Autodesk Inventor part; units mm, degrees
ref_plane "YZ Plane" through (0, 0, 0) normal (1, 0, 0) x (0, 1, 0)
ref_plane "XZ Plane" through (0, 0, 0) normal (0, 1, 0) x (-1, 0, 0)
ref_plane "XY Plane" through (0, 0, 0) normal (0, 0, 1) x (1, 0, 0)
sketch "Sketch1" plane through (0, 0, 0) normal (0, 0, 1) x (1, 0, 0)
  line L0 (0, 0) -> (14, 0)
  line L1 (14, 0) -> (14, -14)
  line L2 (14, -14) -> (0, -14)
  line L3 (0, -14) -> (0, 0)
  dimension "d0" = 14
  dimension "d1" = 14
extrude "Extrusion1" add sketch "Sketch1" against normal blind 22
sketch "Sketch2" plane through (0, 0, 0) normal (0, 0, 1) x (1, 0, 0)
  line L0 (2, -2) -> (12, -2)
  line L1 (12, -2) -> (12, -22)
  line L2 (12, -22) -> (2, -22)
  line L3 (2, -22) -> (2, -2)
  point P0 (0, 0)
  dimension "d4" = 10
  dimension "d5" = 20
extrude "Extrusion2" cut sketch "Sketch2" against normal blind 20
sketch "Sketch5" plane through (0, -14, 0) normal (-1, 0, 0) x (0, 0, 1)
  line L0 (-13, 12) -> (-18, 12)
  line L1 (-18, 12) -> (-18, -8)
  line L2 (-18, -8) -> (-13, -8)
  line L3 (-13, -8) -> (-13, 12)
  point P0 (0, 14)
  dimension "d11" = 5
  dimension "d12" = 20
extrude "Extrusion4" cut sketch "Sketch5" against normal blind 2
properties part number "housing_v03"
Read the model definition and answer for the solid it produces. Units are mm, in the model's axes. A direction names the side the tool comes from. Round coordinates to 2 decimals unless told otherwise and drop trailing zeros. Write each loop counter-clockwise with the first axis right and the second up, starting at its lowest first coordinate (ties: lowest second). Pieces come first, ordered by that corner, then holes. Notation, with made-up numbers: (45.5, 70.5) - (51.5, 70.5) arc R27 cw to (51.5, 102.5) - close; hole circle Ø2 at (-2, -21). An arc over 180 degrees is marked (long way). Use CSV: the item, a comma, the result in double quotes.
Q1. This flat-tipped pin is pushed along its axis until it touches: pin 1 Ø3.5 at (x, z) = (7.5, -9) entering from -Y. Where does it stop, or does it pass through?
Values:
pin 1,"stops at y = -2"
Q2. A tool of negligible diameter and unlimited length cuts with its end or side. For faces 1 (the flat face through (1, -8, -13)), 2 (the flat face through (14, -7, -11)), 3 (the flat face through (2, -8, -6)), from which of +Z, -Z, +X, -X, +Y, -Y can it reach the whole face along a straight path? Write none if from no direction.
Values:
face 1,"-X, -Y"
face 2,"+Z, -Z, +X, +Y, -Y"
face 3,"+Z, -Y"
Q3. Find section C-C, the plane x = 8. Write down the section's boundary in (y, z), then the cut area to 3 significant figures.
Values:
outline,"(-14, -22) - (0, -22) - (0, 0) - (-2, 0) - (-2, -20) - (-14, -20) - close"
area,"68.0 mm²"
Q4. Find section D-D, the plane z = -14. Write down the section's boundary in (x, y), then the cut area to 3 significant figures.
Values:
outline,"(0, -2) - (12, -2) - (12, -14) - (14, -14) - (14, 0) - (0, 0) - close"
area,"52.0 mm²"
Q5. Find section B-B, the plane z = -5.5. Write down the section's boundary in (x, y), then the cut area to 3 significant figures.
Values:
outline,"(0, -14) - (2, -14) - (2, -2) - (12, -2) - (12, -14) - (14, -14) - (14, 0) - (0, 0) - close"
area,"76.0 mm²"
Q6. Find section A-A, the plane y = -3.25. Write down the section's boundary in (x, z).
Values:
outline,"(0, -22) - (14, -22) - (14, 0) - (12, 0) - (12, -20) - (2, -20) - (2, -18) - (0, -18) - close; (0, -13) - (2, -13) - (2, 0) - (0, 0) - close"
Q7. Determine the mould class of faces 4 (the flat face through (12.2, -14, -14.2)), 5 (the flat face through (0, -7, -11)), 6 (the flat face through (7, -2, -10)) for opening direction X: +X half, -X half, draft (parallel to the pull), parting line (faces both ways), or undercut.
Values:
face 4,"draft"
face 5,"-X half"
face 6,"undercut"
Q8. Straight lines are drawn through the part: line 1 along Z through (x, y) = (0.75, -4.5); line 2 along X through (y, z) = (-7, -10.75); line 3 along Z through (x, y) = (7, -12.25). For each, find the intervals that lie inside material, in ascending order.
Values:
line 1,"z = -22 to -18, -13 to 0"
line 2,"x = 0 to 2, 12 to 14"
line 3,"z = -22 to -20"
